Read the model definition and answer for the solid it produces. Units are mm, in the model's axes. A direction names the side the tool comes from. Give positions to 0.01 mm unless a question says otherwise; leave off trailing zeros. Loops run counter-clockwise (first coordinate to the right, second up) from the corner with the lowest first, then second, coordinate; pieces in that order, holes last. Notation, with made-up numbers: (39, -39.5) -> (69, -39.5) arc R17 ccw to (69, -28.5) -> close; hole circle Ø4 at (37.25, 78). An arc over 180 degrees is marked (long way). One line per item, written item: value. Start each with the question number.
from build123d import *

# Parameters (mm, degrees)
ESQUISSE1_W        = 70
ESQUISSE1_H        = 62
BOSS_EXTRU_1_DEPTH = 2
ESQUISSE2_W        = 35
ESQUISSE2_H        = 24
BOSS_EXTRU_2_DEPTH = 15
ESQUISSE3_W        = 39
ESQUISSE3_H        = 3
BOSS_EXTRU_3_DEPTH = 22
ESQUISSE4_W        = 48
ESQUISSE4_H        = 3
BOSS_EXTRU_4_DEPTH = 10
ESQUISSE5_R        = 5
BOSS_EXTRU_5_DEPTH = 190


with BuildPart() as part:
    # Esquisse1 → Boss.-Extru.1 (new body)
    with BuildSketch(Plane.XY):
        Rectangle(ESQUISSE1_W, ESQUISSE1_H)
    extrude(amount=BOSS_EXTRU_1_DEPTH)

    # Esquisse2 → Boss.-Extru.2 (add)
    with BuildSketch(Plane.XY):
        with Locations((-17.5, 3)):
            Rectangle(ESQUISSE2_W, ESQUISSE2_H)
    extrude(amount=BOSS_EXTRU_2_DEPTH)

    # Esquisse3 → Boss.-Extru.3 (add)
    with BuildSketch(Plane.XY):
        with Locations((15.5, -19.5)):
            Rectangle(ESQUISSE3_W, ESQUISSE3_H)
    extrude(amount=BOSS_EXTRU_3_DEPTH)

    # Esquisse4 → Boss.-Extru.4 (add)
    with BuildSketch(Plane.XY):
        with Locations((11, 26.5)):
            Rectangle(ESQUISSE4_W, ESQUISSE4_H)
    extrude(amount=BOSS_EXTRU_4_DEPTH)

    # Esquisse5 → Boss.-Extru.5 (add)
    with BuildSketch(Plane.ZY.offset(35)):
        with Locations(Location((8.5, 8, 0), (0, 0, 90))):
            Circle(ESQUISSE5_R)
    extrude(amount=BOSS_EXTRU_5_DEPTH)


solid = part.part
Item 1: Section B-B, the plane z = 19.5 is taken. Determine the outline of the cut face in (x, y).
Item 2: For faces 4 (the flat face through (15, -21, 12)), 5 (the flat face through (0, 3, 8)), 6 (the flat face through (15, -18, 12)), determine the directions among +Z, -Z, +X, -X, +Y, -Y from which every point of the face is accessible in a straight line to the end or side of a thin tool.
Item 3: Consider L1, parallel to Y at x = 1, z = 4.75; L2, parallel to X at y = -18.5, z = 10.5; L3, parallel to X at y = 22, z = 1.75. Determine where each line is inside the solid, lowest interval first. Write a range as [from, to].
Item 4: Flat-ended cylindrical pins translate along their axes: pin 1 (5 mm diameter, centred on y = -20, z = 6, fed in from -X); pin 2 (0.9 mm diameter, centred on x = 20.5, y = 26, fed in from +Z); pin 3 (19 mm diameter, centred on x = -14, y = 8, fed in from +Z). Find the tip coordinate at first contact, or state that the pin passes through.
Item 5: Determine the mould class of faces 1 (the flat face through (35, -2, 1)), 2 (the flat face through (11, 25, 6)), 3 (the cylindrical face through (-128.67, 12.77, 7)) for opening direction Y: pulls with the +Y half, pulls with the -Y half, needs draft (parallel to the pull), parting line crosses it, or undercut.
Item 6: Section A-A, the plane y = 8 is taken. Determine the outline of the cut face in (x, z), plus the area to 4 significant figures.
Item 7: Section C-C, the plane x = -127 is taken. Determine the outline of the cut face in (y, z).
Computed values:
1. outline: (-4, -21) -> (35, -21) -> (35, -18) -> (-4, -18) -> close
2. face 4: +Z, +X, -X, -Y
2. face 5: +Z, +X
2. face 6: +Z, +X, -X
3. L1: [-21, -18], [25, 28]
3. L2: [-4, 35]
3. L3: [-35, 35]
4. pin 1: x = -4
4. pin 2: z = 10
4. pin 3: z = 15
5. face 1: needs draft
5. face 2: undercut
5. face 3: parting line crosses it
6. outline: (-225, 3.5) -> (-35, 3.5) -> (-35, 0) -> (35, 0) -> (35, 2) -> (0, 2) -> (0, 15) -> (-35, 15) -> (-35, 13.5) -> (-225, 13.5) -> close
6. area: 2,495 mm²
7. outline: circle Ø10 at (8, 8.5)
